```python
from build123d import *

# Parameters (mm, degrees)
SKETCH_W        = 40
SKETCH_H        = 96.5
PAD_DEPTH       = 2
SKETCH001_R     = 1.7
SKETCH001_R_2   = 1.5
SKETCH001_R_3   = 2.5
SKETCH001_R_4   = 1.8
SKETCH001_W     = 11
SKETCH001_H     = 41
POCKET_DEPTH    = 5
FILLET_R        = 2
FILLET001_R     = 2
SKETCH004_W     = 20
SKETCH004_H     = 3
PAD002_DEPTH    = 15
SKETCH005_R     = 1.6
POCKET002_DEPTH = 5


with BuildPart() as part:
    # Sketch → Pad (new body)
    with BuildSketch(Plane.XY):
        Rectangle(SKETCH_W, SKETCH_H)
    extrude(amount=PAD_DEPTH)

    # Sketch001 (on Face6 of Pad) → Pocket (cut)
    with BuildSketch(Plane.XY.offset(2)):
        with Locations((-16.5, 44.95)):
            Circle(SKETCH001_R)
        with Locations((16.5, 44.95)):
            Circle(SKETCH001_R)
        with Locations((-16.5, -44.95)):
            Circle(SKETCH001_R)
        with Locations((16.5, -44.95)):
            Circle(SKETCH001_R)
        with Locations((-10.86, 38.85)):
            Circle(SKETCH001_R_2)
        with Locations((-10.86, -7.75)):
            Circle(SKETCH001_R_2)
        with Locations((-2.5, -14.75)):
            Circle(SKETCH001_R_3)
        with Locations((-15, -27.25)):
            Circle(SKETCH001_R_4)
        with Locations((10, -27.25)):
            Circle(SKETCH001_R_4)
        with Locations((9.220326, 38.85)):
            Circle(SKETCH001_R_2)
        with Locations((9.220326, -7.75)):
            Circle(SKETCH001_R_2)
        with Locations((-10.68, 15.55)):
            Rectangle(SKETCH001_W, SKETCH001_H)
        with Locations((9.400326, 15.55)):
            Rectangle(SKETCH001_W, SKETCH001_H)
    extrude(amount=-POCKET_DEPTH, mode=Mode.SUBTRACT)

    # Fillet
    fillet_edges = [part.edges().sort_by_distance(p)[0] for p in [
        (-20, 48.25, 1),
    ]]
    fillet(fillet_edges, radius=FILLET_R)

    # Fillet001
    fillet001_edges = [part.edges().sort_by_distance(p)[0] for p in [
        (20, 48.25, 1),
    ]]
    fillet(fillet001_edges, radius=FILLET001_R)

    # Sketch004 → Pad002 (join)
    with BuildSketch(Plane.XY.offset(2)):
        with Locations((0, -46.75)):
            Rectangle(SKETCH004_W, SKETCH004_H)
    extrude(amount=PAD002_DEPTH)

    # Sketch005 (on Face40 of Pad002) → Pocket002 (cut)
    with BuildSketch(Plane.XZ.offset(48.25)):
        with Locations((0, 10.420713)):
            Circle(SKETCH005_R)
    extrude(amount=-POCKET002_DEPTH, mode=Mode.SUBTRACT)


solid = part.part
```
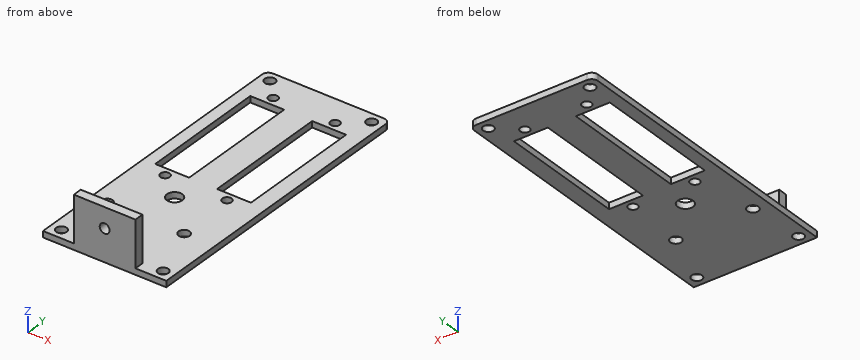
Design review of the part built by this model. Coordinates are the model's own, in mm. Coordinates: 2 decimals unless noted, no trailing zeros. Write each loop counter-clockwise with the first axis right and the second up, starting at its lowest first coordinate (ties: lowest second). Pieces come first, ordered by that corner, then holes.
1) Add section B-B (x = 16.5). Write out the cut boundary in (y, z).
2) To check wall thickness, follow L1, parallel to X at y = 22.5, z = 1; L2, parallel to Z at x = 14, y = -28; L3, parallel to Y at x = -2, z = 5.5. State the ranges of each line that lie inside material, in increasing order.
3) Insertion check: pin 1 (4 mm diameter, centred on x = -10.86, y = -7.75, fed in from +Z); pin 2 (3 mm diameter, centred on x = -7, z = 7.5, fed in from +Y); pin 3 (3.5 mm diameter, centred on y = -46.5, z = 10, fed in from +X). Each pin has a flat end and moves straight along its axis. Give the tip position at first contact, or say it passes through.
4) Add section C-C (x = -10.86). Write out the cut boundary in (y, z).
5) Add section A-A (y = -27.25). Write out the cut boundary in (x, z), plus the area to 3 significant figures.
Check result:
1. outline: (-48.25, 0) - (-46.65, 0) - (-46.65, 2) - (-48.25, 2) - close; (-43.25, 0) - (43.25, 0) - (43.25, 2) - (-43.25, 2) - close; (46.65, 0) - (48.25, 0) - (48.25, 2) - (46.65, 2) - close
2. L1: x = -20 to -16.18, -5.18 to 3.9, 14.9 to 20
2. L2: z = 0 to 2
2. L3: y = -48.25 to -45.25
3. pin 1: stops at z = 2
3. pin 2: stops at y = -45.25
3. pin 3: stops at x = 10
4. outline: (-48.25, 0) - (-9.25, 0) - (-9.25, 2) - (-48.25, 2) - close; (-6.25, 0) - (-4.95, 0) - (-4.95, 2) - (-6.25, 2) - close; (36.05, 0) - (37.35, 0) - (37.35, 2) - (36.05, 2) - close; (40.35, 0) - (48.25, 0) - (48.25, 2) - (40.35, 2) - close
5. outline: (-20, 0) - (-16.8, 0) - (-16.8, 2) - (-20, 2) - close; (-13.2, 0) - (8.2, 0) - (8.2, 2) - (-13.2, 2) - close; (11.8, 0) - (20, 0) - (20, 2) - (11.8, 2) - close
5. area: 65.6 mm2
